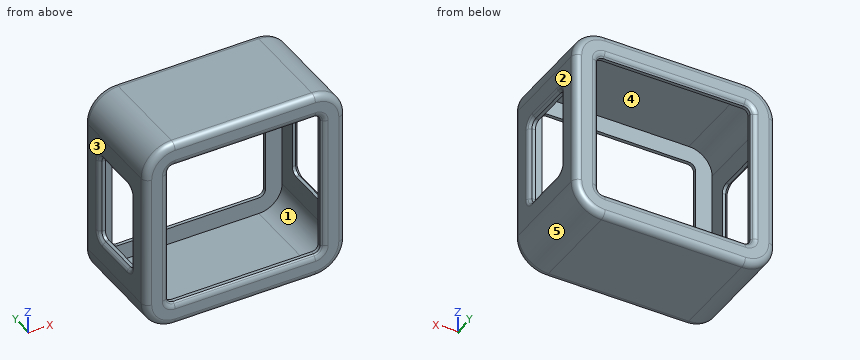
from build123d import *

# Parameters (mm, degrees)
FILLET6_TOP_FACE_R                     = 1
CUT_EXTRUDE1_SIDE_APERTURE_REACH       = 41.369
SKETCH3_W                              = 13.2
SKETCH3_H                              = 7.3
MIRROR11_COPY_1_REACH                  = 41.369
MIRROR11_COPY_1_SKETCH_W               = 13.2
MIRROR11_COPY_1_SKETCH_H               = 7.3
FILLET6_TOP_FACE_OF_MIRROR11_R         = 1
FILLET4_SIDE_APERTURE_INSIDE_CORNERS_R = 1
CHAMFER1_SIDE_APERTURE_SIZE            = 0.5
FILLET5_SIDE_APERTURE_R                = 0.5


with BuildPart() as part:
    # Sweep1: sweep along a path in Sketch2
    with BuildLine(Plane(origin=(0, 5.050213041, 0), x_dir=(1, 0, 0), z_dir=(0, 1, 0))) as sweep1_path:
        Line((1.5, 0), (1.5, 20))
        ThreePointArc((1.5, 20), (0.474873734, 22.474873734), (-2, 23.5))
        Line((-2, 23.5), (-23, 23.5))
        ThreePointArc((-23, 23.5), (-25.474873734, 22.474873734), (-26.5, 20))
        Line((-26.5, 20), (-26.5, 0))
        ThreePointArc((-26.5, 0), (-25.474873734, -2.474873734), (-23, -3.5))
        Line((-23, -3.5), (-2, -3.5))
        ThreePointArc((-2, -3.5), (0.474873734, -2.474873734), (1.5, 0))
    # Sketch1 → Sweep1 (sweep)
    with BuildSketch(Plane.XY):
        Polygon((1.5, 6.050213041), (1.5, -0.8), (2.5, -0.8), (2.5, 7.050213041), (-0.5, 7.050213041), (-1, 6.550213041), (-1, 6.050213041), align=None)
    sweep1 = sweep(path=sweep1_path.line)

    # Fillet6 (top face)
    fillet6_top_face_edges = [part.edges().sort_by_distance(p)[0] for p in [
        (-12.5, 7.050213041, -24.5),
        (-12.5, 7.050213041, -21.5),
        (-26.181980515, 7.050213041, -23.181980515),
        (-24.060660172, 7.050213041, -21.060660172),
        (-27.5, 7.050213041, -10),
        (-24.5, 7.050213041, -10),
        (-26.181980515, 7.050213041, 3.181980515),
        (-24.060660172, 7.050213041, 1.060660172),
        (-12.5, 7.050213041, 4.5),
        (-12.5, 7.050213041, 1.5),
        (1.181980515, 7.050213041, 3.181980515),
        (-0.939339828, 7.050213041, 1.060660172),
        (2.5, 7.050213041, -10),
        (-0.5, 7.050213041, -10),
        (1.181980515, 7.050213041, -23.181980515),
        (-0.939339828, 7.050213041, -21.060660172),
    ]]
    fillet(fillet6_top_face_edges, radius=FILLET6_TOP_FACE_R)

    # Sketch3 → Cut-Extrude1 (side aperture) (cut, up to next)
    with BuildSketch(Plane(origin=(2.5, 0, 0), x_dir=(0, 0, -1), z_dir=(1, 0, 0)), mode=Mode.PRIVATE) as cut_extrude1_side_aperture_sk1:
        with Locations((10, -0.249786959)):
            Rectangle(SKETCH3_W, SKETCH3_H)
    cut_extrude1_side_aperture_tool1 = extrude(cut_extrude1_side_aperture_sk1.sketch, amount=-CUT_EXTRUDE1_SIDE_APERTURE_REACH, mode=Mode.PRIVATE) & part.part
    cut_extrude1_side_aperture = cut_extrude1_side_aperture_tool1.solids().sort_by_distance((2.5, -0.249787, -10))[0]
    add(cut_extrude1_side_aperture, mode=Mode.SUBTRACT)

    # Mirror6: Cut-Extrude1 (side aperture) across plane
    add(cut_extrude1_side_aperture.mirror(Plane.ZY.offset(12.5)), mode=Mode.SUBTRACT)

    # Mirror11: Sweep1, Cut-Extrude1 (side aperture) across plane
    add(sweep1.mirror(Plane.ZX.offset(-0.8)))
    add(cut_extrude1_side_aperture.mirror(Plane.ZX.offset(-0.8)), mode=Mode.SUBTRACT)

    # Mirror11 copy 1 sketch → Mirror11 copy 1 (cut, up to next)
    with BuildSketch(Plane(origin=(-27.5, -1.6, 0), x_dir=(0, 0, -1), z_dir=(-1, 0, 0)), mode=Mode.PRIVATE) as mirror11_copy_1_sk1:
        with Locations((10, -0.249786959)):
            Rectangle(MIRROR11_COPY_1_SKETCH_W, MIRROR11_COPY_1_SKETCH_H)
    mirror11_copy_1_tool1 = extrude(mirror11_copy_1_sk1.sketch, amount=-MIRROR11_COPY_1_REACH, mode=Mode.PRIVATE) & part.part
    add(mirror11_copy_1_tool1.solids().sort_by_distance((-27.5, -1.350213, -10))[0], mode=Mode.SUBTRACT)

    # Fillet6 (top face) of Mirror11
    fillet6_top_face_of_mirror11_edges = [part.edges().sort_by_distance(p)[0] for p in [
        (-12.5, -8.650213041, -24.5),
        (-12.5, -8.650213041, -21.5),
        (-26.181980515, -8.650213041, -23.181980515),
        (-24.060660172, -8.650213041, -21.060660172),
        (-27.5, -8.650213041, -10),
        (-24.5, -8.650213041, -10),
        (-26.181980515, -8.650213041, 3.181980515),
        (-24.060660172, -8.650213041, 1.060660172),
        (-12.5, -8.650213041, 4.5),
        (-12.5, -8.650213041, 1.5),
        (1.181980515, -8.650213041, 3.181980515),
        (-0.939339828, -8.650213041, 1.060660172),
        (2.5, -8.650213041, -10),
        (-0.5, -8.650213041, -10),
        (1.181980515, -8.650213041, -23.181980515),
        (-0.939339828, -8.650213041, -21.060660172),
    ]]
    fillet(fillet6_top_face_of_mirror11_edges, radius=FILLET6_TOP_FACE_OF_MIRROR11_R)

    # Fillet4 (side aperture inside corners)
    fillet4_side_aperture_inside_corners_edges = [part.edges().sort_by_distance(p)[0] for p in [
        (2, 3.400213041, -16.6),
        (2, 3.400213041, -3.4),
        (-27, 3.400213041, -16.6),
        (-27, 3.400213041, -3.4),
        (2, -5.000213041, -3.4),
        (2, -5.000213041, -16.6),
        (-27, -5.000213041, -3.4),
        (-27, -5.000213041, -16.6),
    ]]
    fillet(fillet4_side_aperture_inside_corners_edges, radius=FILLET4_SIDE_APERTURE_INSIDE_CORNERS_R)

    # Chamfer1 (side aperture)
    chamfer1_side_aperture_edges = [part.edges().sort_by_distance(p)[0] for p in [
        (-27.5, -0.8, -16.6),
        (-27.5, 3.400213041, -10),
        (-27.5, -5.000213041, -10),
        (-27.5, -0.8, -3.4),
        (2.5, -5.000213041, -10),
        (2.5, -0.8, -3.4),
        (2.5, -0.8, -16.6),
        (2.5, 3.400213041, -10),
        (-27.5, 3.107319822, -16.307106781),
        (-27.5, -4.707319822, -16.307106781),
        (-27.5, 3.107319822, -3.692893219),
        (-27.5, -4.707319822, -3.692893219),
        (2.5, -4.707319822, -3.692893219),
        (2.5, -4.707319822, -16.307106781),
        (2.5, 3.107319822, -3.692893219),
        (2.5, 3.107319822, -16.307106781),
    ]]
    chamfer(chamfer1_side_aperture_edges, length=CHAMFER1_SIDE_APERTURE_SIZE)

    # Fillet5 (side aperture)
    fillet5_side_aperture_edges = [part.edges().sort_by_distance(p)[0] for p in [
        (-27.5, -0.8, -17.1),
        (-27.5, 3.460873213, -16.660660172),
        (-27.5, -5.060873213, -16.660660172),
        (-27.5, 3.900213041, -10),
        (-27.5, -5.500213041, -10),
        (-27.5, 3.460873213, -3.339339828),
        (-27.5, -5.060873213, -3.339339828),
        (-27.5, -0.8, -2.9),
        (2.5, -0.8, -2.9),
        (2.5, 3.460873213, -3.339339828),
        (2.5, 3.900213041, -10),
        (2.5, 3.460873213, -16.660660172),
        (2.5, -0.8, -17.1),
        (2.5, -5.060873213, -3.339339828),
        (2.5, -5.060873213, -16.660660172),
        (2.5, -5.500213041, -10),
    ]]
    fillet(fillet5_side_aperture_edges, radius=FILLET5_SIDE_APERTURE_R)


solid = part.part
Source: CAD feature listing. Evaluate the final solid. Frame: model axes, mm. Face numbers are marked on the shaded views. A direction names the side the tool comes from. Round coordinates to 2 decimals unless told otherwise and drop trailing zeros. Order: outer loops, then holes, each group sorted by start corner. A loop starts at its lowest first (then second) coordinate and runs counter-clockwise, first axis right, second up. Notation, with made-up numbers: (88.25, 34) -> (124.25, 34) arc R21 cw to (124.25, 71) -> close; hole circle Ø11 at (-16.75, 22.25). An arc over 180 degrees is marked (long way). Answer as CSV lines item,"result".
Item 1: Section B-B, the plane x = -14.5. Return loops of the section in (y, z).
A:
outline,"(-8.65, -23.5) arc R1 ccw to (-7.65, -24.5) -> (6.05, -24.5) arc R1 ccw to (7.05, -23.5) -> (7.05, -21.91) arc R1 ccw to (6.76, -21.21) -> (6.55, -21) -> (6.05, -21) -> (6.05, -23.5) -> (-7.65, -23.5) -> (-7.65, -21) -> (-8.15, -21) -> (-8.36, -21.21) arc R1 ccw to (-8.65, -21.91) -> close; (-8.65, 1.91) arc R1 ccw to (-8.36, 1.21) -> (-8.15, 1) -> (-7.65, 1) -> (-7.65, 3.5) -> (6.05, 3.5) -> (6.05, 1) -> (6.55, 1) -> (6.76, 1.21) arc R1 ccw to (7.05, 1.91) -> (7.05, 3.5) arc R1 ccw to (6.05, 4.5) -> (-7.65, 4.5) arc R1 ccw to (-8.65, 3.5) -> close"
Item 2: Reachability of the marked faces 1 and 2 from +Z, -Z, +X, -X, +Y, -Y: full face, straight path, thin tool, end or side. Return the list, or none.
A:
face 1,"none"
face 2,"+Z, -Z, +X, +Y, -Y"
Item 3: Pin query (flat end, axial travel): pin 1 Ø0.6 at (x, z) = (2, -11) entering from -Y; pin 2 Ø0.6 at (x, y) = (2, -1) entering from -Z. Return the tip coordinate at first contact, or that it passes through.
A:
pin 1,"y = -8.63"
pin 2,"z = -22.56"
Item 4: Line query: L1, parallel to Z at x = -20, y = -3.25; L2, parallel to X at y = 6, z = -12.5; L3, parallel to Z at x = -24, y = 3.25. Output: solid intervals per line, ascending.
A:
L1,"-24.5 to -23.5, 3.5 to 4.5"
L2,"-27.5 to -26.5, 1.5 to 2.5"
L3,"-24.39 to -23.35, 3.35 to 4.39"
Item 5: Section C-C, the plane z = -19.5. Return loops of the section in (x, y).
A:
outline,"(-27.5, -7.65) arc R1 ccw to (-26.5, -8.65) -> (-24.91, -8.65) arc R1 ccw to (-24.21, -8.36) -> (-24, -8.15) -> (-24, -7.65) -> (-26.5, -7.65) -> (-26.5, 6.05) -> (-24, 6.05) -> (-24, 6.55) -> (-24.21, 6.76) arc R1 ccw to (-24.91, 7.05) -> (-26.5, 7.05) arc R1 ccw to (-27.5, 6.05) -> close; (-1, -8.15) -> (-0.79, -8.36) arc R1 ccw to (-0.09, -8.65) -> (1.5, -8.65) arc R1 ccw to (2.5, -7.65) -> (2.5, 6.05) arc R1 ccw to (1.5, 7.05) -> (-0.09, 7.05) arc R1 ccw to (-0.79, 6.76) -> (-1, 6.55) -> (-1, 6.05) -> (1.5, 6.05) -> (1.5, -7.65) -> (-1, -7.65) -> close"
Item 6: Pull-direction query (X, two-part tool) for the marked faces 3, 4 and 5; classes: pulls with the +X half, pulls with the -X half, needs draft (parallel to the pull), parting line crosses it, or undercut.
A:
face 3,"pulls with the -X half"
face 4,"undercut"
face 5,"pulls with the +X half"
Item 7: Section D-D, the plane y = -7. Return loops of the section in (x, z), plus the area to 3 significant figures.
A:
outline,"(-27.5, -20) arc R4.5 ccw to (-23, -24.5) -> (-2, -24.5) arc R4.5 ccw to (2.5, -20) -> (2.5, 0) arc R4.5 ccw to (-2, 4.5) -> (-23, 4.5) arc R4.5 ccw to (-27.5, 0) -> close; hole (-26.5, -20) arc R3.5 ccw to (-23, -23.5) -> (-2, -23.5) arc R3.5 ccw to (1.5, -20) -> (1.5, 0) arc R3.5 ccw to (-2, 3.5) -> (-23, 3.5) arc R3.5 ccw to (-26.5, 0) -> close"
area,"107 mm²"
